Could you check a few things on this model? Use its own coordinates, in mm. Face numbers are marked on the shaded views. A direction names the side the tool comes from. Give positions to 0.01 mm unless a question says otherwise; leave off trailing zeros. Loops run counter-clockwise (first coordinate to the right, second up) from the corner with the lowest first, then second, coordinate; pieces in that order, holes last. Notation, with made-up numbers: M 16,-1 L 54,-1 A14 ccw 54,6 Z; hole C 4.5,52.25 d11. An arc over 180 degrees is marked long. Answer in a Markdown table with one row per item. Add a question column.
```python
from build123d import *

# Parameters (mm, degrees)
SKETCH1_R           = 7.5
BOSS_EXTRUDE1_DEPTH = 4
SKETCH4_R           = 7.5
BOSS_EXTRUDE4_DEPTH = 8
BOSS_EXTRUDE4_TAPER = 20
SKETCH5_R           = 1.5
CUT_EXTRUDE2_DEPTH  = 17.015617547
SKETCH6_R           = 3
CUT_EXTRUDE3_DEPTH  = 9
SKETCH7_R           = 1.5
CUT_EXTRUDE4_DEPTH  = 23.505555034
SKETCH8_R           = 1.5
CUT_EXTRUDE5_DEPTH  = 23.505555034


with BuildPart() as part:
    # Sketch1 → Boss-Extrude1 (new body)
    with BuildSketch(Plane(origin=(0, 0, 0), x_dir=(1, 0, 0), z_dir=(0, 1, 0))):
        with Locations(Location((0, 0, 0), (0, 0, 270))):
            Circle(SKETCH1_R)
    extrude(amount=BOSS_EXTRUDE1_DEPTH)

    # Sketch4 → Boss-Extrude4 (add)
    with BuildSketch(Plane(origin=(0, 4, 0), x_dir=(1, 0, 0), z_dir=(0, 1, 0))):
        with Locations(Location((0, 0, 0), (0, 0, 270))):
            Circle(SKETCH4_R)
    extrude(amount=BOSS_EXTRUDE4_DEPTH, taper=BOSS_EXTRUDE4_TAPER)

    # Sketch5 → Cut-Extrude2 (cut, through all)
    with BuildSketch(Plane(origin=(0, 0, 0), x_dir=(-1, 0, 0), z_dir=(0, -1, 0))):
        with Locations(Location((0, 0, 0), (0, 0, 90))):
            Circle(SKETCH5_R)
    extrude(amount=-CUT_EXTRUDE2_DEPTH, mode=Mode.SUBTRACT)

    # Sketch6 → Cut-Extrude3 (cut)
    with BuildSketch(Plane(origin=(0, 12, 0), x_dir=(1, 0, 0), z_dir=(0, 1, 0))):
        with Locations(Location((0, 0, 0), (0, 0, 270))):
            Circle(SKETCH6_R)
    extrude(amount=-CUT_EXTRUDE3_DEPTH, mode=Mode.SUBTRACT)

    # Sketch7 → Cut-Extrude4 (cut, through all)
    with BuildSketch(Plane.XY.offset(10)):
        with Locations((0, 8)):
            Circle(SKETCH7_R)
    extrude(amount=-CUT_EXTRUDE4_DEPTH, mode=Mode.SUBTRACT)

    # Sketch8 → Cut-Extrude5 (cut, through all)
    with BuildSketch(Plane.XY.offset(10)):
        with Locations((0, 7)):
            Circle(SKETCH8_R)
    extrude(amount=-CUT_EXTRUDE5_DEPTH, mode=Mode.SUBTRACT)


solid = part.part
```
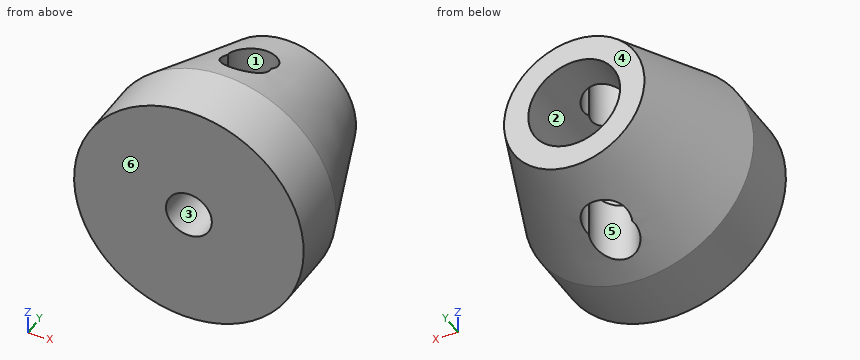
Item 1: Suppose I cut it at A-A (z = 0). List the corners of the cut face in (x, y) for me.
Item 2: Suppose I cut it at B-B (y = 8). List the corners of the cut face in (x, z) for me, then the cut area to 3 significant figures.
Item 3: For the marked faces 1 and 2, which set-ups out of +Z, -Z, +X, -X, +Y, -Y let a thin tool reach every point of the face, with its end or its side?
Item 4: Suppose I cut it at C-C (y = 1.5). List the corners of the cut face in (x, z) for me.
Item 5: Suppose I cut it at D-D (x = 0). Give the number of separate pieces and of enclosed holes in the cut face, then the cut area to 3 significant figures.
Item 6: I need wall thicknesses on L1, parallel to X at y = 1.8, z = 0; L2, parallel to X at y = 5.5, z = 0; L3, parallel to Y at x = 0, z = 3.65. Which ranges of each line are inside material? Lowest first, please.
Item 7: For P1, Ø4, axis at x = -4, y = 6.5, coming from the -Z side; P2, Ø5, axis at x = 0, y = 7, coming from the -Z side; P3, Ø4, axis at x = -4.5, y = 4.5, coming from the +Z side; P4, Ø2.5, axis at x = 0, y = 8, coming from the -Z side, each with a flat end and sliding along its axis, tell me the tip position at first contact or that it passes through.
Item 8: If we mould it in two halves opening along Y, with no side actions, what happens to the marked faces 3, 4, 5 and 6? For each: +Y half, -Y half, draft (parallel to the pull), parting line (faces both ways), or undercut.
Values found:
| question | item | result |
|---|---|---|
| 1 | outline | M -7.5,0 L -1.5,0 L -1.5,3 L -3,3 L -3,12 L -4.59,12 L -7.5,4 Z; M 1.5,0 L 7.5,0 L 7.5,4 L 4.59,12 L 3,12 L 3,3 L 1.5,3 Z |
| 2 | outline | M -1.5,-5.86 L -1.5,-2.6 A3 cw -1.5,2.6 L -1.5,5.86 A6.04 ccw Z; M 1.5,-5.86 A6.04 ccw 1.5,5.86 L 1.5,2.6 A3 cw 1.5,-2.6 Z |
| 2 | area | 67.8 mm² |
| 3 | face 1 | +Z, -Z |
| 3 | face 2 | +Y |
| 4 | outline | C 0,0 d15; hole C 0,0 d3 |
| 5 | separate pieces | 4 |
| 5 | enclosed holes | 0 |
| 5 | area | 67.9 mm² |
| 6 | L1 | -7.5 to -1.5, 1.5 to 7.5 |
| 6 | L2 | -6.95 to -3, 3 to 6.95 |
| 6 | L3 | 0 to 5.5, 9.5 to 12 |
| 7 | P1 | z = -6.62 |
| 7 | P2 | z = -7.32 |
| 7 | P3 | z = 7.05 |
| 7 | P4 | through |
| 8 | face 3 | draft |
| 8 | face 4 | +Y half |
| 8 | face 5 | undercut |
| 8 | face 6 | -Y half |
